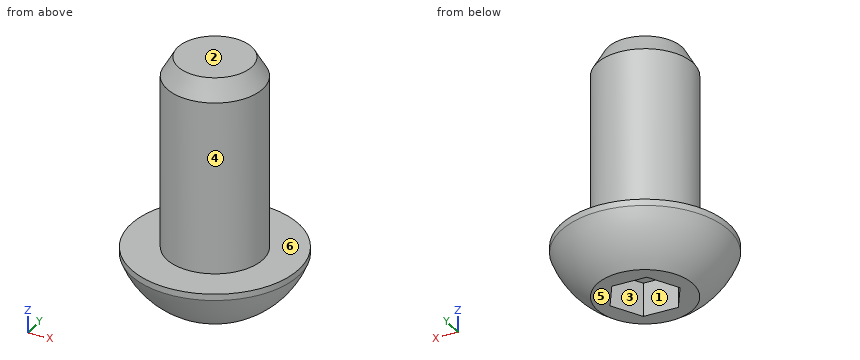
```python
from build123d import *

# Parameters (mm, degrees)
CUT_EXTRUDE1_DEPTH  = 2.2225
SKETCH3_R           = 3.175
BOSS_EXTRUDE1_DEPTH = 12.7
CHAMFER1_SIZE       = 1.27
CHAMFER1_SIZE2      = 0.733234842


with BuildPart() as part:
    # Sketch1 → Revolve1 (revolve)
    with BuildSketch(Plane(origin=(0, 0, 0), x_dir=(1, 0, 0), z_dir=(0, 1, 0))):
        with BuildLine():
            Line((5.549899963, -3.3528), (5.549899963, -2.933699945))
            ThreePointArc((5.549899963, -2.933699945), (4.602457888, -1.27255785), (3.174999986, 0))
            Line((3.174999986, 0), (-1.6e-08, 0))
            Line((-1.6e-08, 0), (-1.6e-08, -3.3528))
            Line((-1.6e-08, -3.3528), (5.549899963, -3.3528))
        make_face()
    revolve(axis=Axis((-1.6e-08, 0, 0), (0, 0, -1)))

    # Sketch2 → Cut-Extrude1 (cut)
    with BuildSketch(Plane(origin=(0, 0, 0), x_dir=(-1, 0, 0), z_dir=(0, 0, -1))):
        Polygon((2.291358881, 0), (1.14567944, 1.984375), (-1.14567944, 1.984375), (-2.291358881, 0), (-1.14567944, -1.984375), (1.14567944, -1.984375), align=None)
    extrude(amount=-CUT_EXTRUDE1_DEPTH, mode=Mode.SUBTRACT)

    # Sketch3 → Boss-Extrude1 (add)
    with BuildSketch(Plane.XY.offset(3.3528)):
        Circle(SKETCH3_R)
    extrude(amount=BOSS_EXTRUDE1_DEPTH)

    # Chamfer1
    chamfer1_edges = [part.edges().sort_by_distance(p)[0] for p in [
        (-3.175, 0, 16.0528),
    ]]
    chamfer1_side = [part.faces().sort_by_distance(p)[0] for p in [
        (-3.175, 0, 9.7028),
    ]]
    chamfer(chamfer1_edges, length=CHAMFER1_SIZE, length2=CHAMFER1_SIZE2, reference=chamfer1_side[0])


solid = part.part
```
Read the model definition and answer for the solid it produces. Units are mm, in the model's axes. Face numbers are marked on the shaded views. A direction names the side the tool comes from. Give positions to 0.01 mm unless a question says otherwise; leave off trailing zeros. Loops run counter-clockwise (first coordinate to the right, second up) from the corner with the lowest first, then second, coordinate; pieces in that order, holes last.
Item 1: The part is cut by section D-D (y = 4.5). Write down the section's boundary in (x, z), and give its area (3 significant figures).
Item 2: For the marked faces 5 and 6, determine the directions among +Z, -Z, +X, -X, +Y, -Y from which every point of the face is accessible in a straight line to the end or side of a thin tool.
Item 3: The mould has two halves that part along X. Classify the marked faces 1, 2, 3 and 4: released by +X, released by -X, zero draft, split by the parting line, or undercut.
Item 4: The part is cut by section C-C (y = -3.5). Write down the section's boundary in (x, z).
Item 5: Each of these flat-tipped pins is pushed along its axis until it touches: pin 1 Ø2.5 at (x, z) = (0.5, 1) entering from -Y; pin 2 Ø0.7 at (x, z) = (-0.5, 1.5) entering from +Y; pin 3 Ø1.5 at (x, y) = (-2, -4) entering from -Z. Where does it stop, or does it pass through?
Item 6: Find the intervals of material crossed by line 1 along Z through (x, y) = (1, -0.25); line 2 along X through (y, z) = (1.25, 1.25); line 3 along X through (y, z) = (-0.75, 7), in increasing order.
Item 7: The part is cut by section B-B (z = 11.5). Write down the section's boundary in (x, y) (3 decimals).
Item 8: The part is cut by section A-A (x = 0). Write down the section's boundary in (y, z) (1 decimal), and give its area (3 significant figures).
Taken from the geometry:
1. outline: (-3.25, 2.93) arc R3.85 ccw to (3.25, 2.93) - (3.25, 3.35) - (-3.25, 3.35) - close
1. area: 10.9 mm2
2. face 5: -Z, +X, -X, +Y, -Y
2. face 6: +Z
3. face 1: undercut
3. face 2: zero draft
3. face 3: undercut
3. face 4: split by the parting line
4. outline: (-4.31, 2.93) arc R4.78 ccw to (4.31, 2.93) - (4.31, 3.35) - (-4.31, 3.35) - close
5. pin 1: stops at y = -5.23
5. pin 2: stops at y = 4.99
5. pin 3: stops at z = 0.39
6. line 1: z = 2.22 to 16.05
6. line 2: x = -4.41 to -1.57, 1.57 to 4.41
6. line 3: x = -3.09 to 3.09
7. outline: circle Ø6.35 at (0, 0)
8. outline: (-5.5, 2.9) arc R5.9 ccw to (-3.2, 0) - (-2, 0) - (-2, 2.2) - (2, 2.2) - (2, 0) - (3.2, 0) arc R5.9 ccw to (5.5, 2.9) - (5.5, 3.4) - (3.2, 3.4) - (3.2, 14.8) - (2.4, 16.1) - (-2.4, 16.1) - (-3.2, 14.8) - (-3.2, 3.4) - (-5.5, 3.4) - close
8. area: 103 mm2
